```python
from build123d import *

# Parameters (mm, degrees)
F0_W     = 151.8794447184
F0_H     = 152.5772064924
F1_DEPTH = 4.318
F2_W     = 130.1674246788
F2_H     = 5.3557232022
F2_H_2   = 7.4514448643
F3_DEPTH = 5.588
F4_W     = 51.2286853045
F4_H     = 29.5729218051
F5_DEPTH = 23.876


with BuildPart() as f1:
    # F0 (on Top) → F1 (new body)
    with BuildSketch(Plane.XY):
        with Locations((0.1162961125, 0)):
            Rectangle(F0_W, F0_H)
    extrude(amount=F1_DEPTH)

    # F2 (on face) → F3 (join)
    with BuildSketch(Plane.XY.offset(4.318)):
        Polygon((-65.2001425624, 63.5701417923), (-65.2001425624, 68.9258649945), (-71.2544471025, 68.9258649945), (-71.2544471025, -70.7887262106), (-65.2001425624, -70.7887262106), (-65.2001425624, -70.5558732152), (-65.2001425624, -63.1044283509), align=None)
        with Locations((-0.116430223, 66.2480033934)):
            Rectangle(F2_W, F2_H)
        Polygon((73.8158747554, 68.9258649945), (64.9672821164, 68.9258649945), (64.9672821164, 63.5701417923), (64.9672821164, -63.1044283509), (64.9672821164, -70.5558732152), (73.8158747554, -70.5558732152), align=None)
        with Locations((-0.116430223, -66.8301507831)):
            Rectangle(F2_W, F2_H_2)
    extrude(amount=F3_DEPTH)

    # F4 (on face) → F5 (join)
    with BuildSketch(Plane.XY.offset(4.318)):
        with Locations((2.0957188681, 10.8278808184)):
            Rectangle(F4_W, F4_H)
    extrude(amount=F5_DEPTH)


solid = f1.part
```
Input: part model. Units: mm. Frame: model coordinates. A direction names the side the tool comes from. Coordinates: 2 decimals unless noted, no trailing zeros. Write each loop counter-clockwise with the first axis right and the second up, starting at its lowest first coordinate (ties: lowest second). Pieces come first, ordered by that corner, then holes.
1) Section B-B on x = 13. Output: boundary loops of the cut face in (y, z).
2) Section A-A on y = 0. Output: boundary loops of the cut face in (x, z).
3) Pin query (flat end, axial travel): pin 1 Ø5 at (x, y) = (-36.5, 31.5) entering from +Z; pin 2 Ø10 at (x, z) = (52.5, 12.5) entering from +Y; pin 3 Ø1.7 at (x, z) = (-68, 8.5) entering from -Y; pin 4 Ø1.5 at (x, y) = (-60.5, -1.5) entering from -Z. Return the tip coordinate at first contact, or that it passes through.
4) Section C-C on z = 19.25. Output: boundary loops of the cut face in (x, y), and give its area (3 significant figures).
5) Set-up query: faces 5 (the flat face through (73.816, -2, 7)), 6 (the flat face through (2, 68.926, 7)), 7 (the flat face through (-71.254, 0, 7)), 8 (the flat face through (64.967, 1, 7)). Return all of +Z, -Z, +X, -X, +Y, -Y with unobstructed straight access to the full face (end or side cutting, diameter ignored); none if empty.
6) Section D-D on y = 36. Output: boundary loops of the cut face in (x, z).
7) Mould query, pull axis X, two halves, no side actions, for faces 1 (the flat face through (-1, 63.57, 7)), 2 (the flat face through (-75.823, -1, 2)), 3 (the flat face through (-1, 1, 0)), 4 (the flat face through (-23.519, 11, 16)). Classes: pulls with the +X half, pulls with the -X half, needs draft (parallel to the pull), parting line crosses it, or undercut.
8) Material intervals for line 1 along X through (y, z) = (24, 9); line 2 along Y through (x, z) = (-7, 4.5); line 3 along X through (y, z) = (30, 6), sorted ascending.
Check result:
1. outline: (-76.29, 0) - (76.29, 0) - (76.29, 4.32) - (68.93, 4.32) - (68.93, 9.91) - (63.57, 9.91) - (63.57, 4.32) - (25.61, 4.32) - (25.61, 28.19) - (-3.96, 28.19) - (-3.96, 4.32) - (-63.1, 4.32) - (-63.1, 9.91) - (-70.56, 9.91) - (-70.56, 4.32) - (-76.29, 4.32) - close
2. outline: (-75.82, 0) - (76.06, 0) - (76.06, 4.32) - (73.82, 4.32) - (73.82, 9.91) - (64.97, 9.91) - (64.97, 4.32) - (27.71, 4.32) - (27.71, 28.19) - (-23.52, 28.19) - (-23.52, 4.32) - (-65.2, 4.32) - (-65.2, 9.91) - (-71.25, 9.91) - (-71.25, 4.32) - (-75.82, 4.32) - close
3. pin 1: stops at z = 4.32
3. pin 2: stops at y = 68.93
3. pin 3: stops at y = -70.79
3. pin 4: stops at z = 0
4. outline: (-23.52, -3.96) - (27.71, -3.96) - (27.71, 25.61) - (-23.52, 25.61) - close
4. area: 1,510 mm2
5. face 5: +Z, +X, +Y, -Y
5. face 6: +Z, +X, -X, +Y
5. face 7: +Z, -X, +Y, -Y
5. face 8: +Z
6. outline: (-75.82, 0) - (76.06, 0) - (76.06, 4.32) - (73.82, 4.32) - (73.82, 9.91) - (64.97, 9.91) - (64.97, 4.32) - (-65.2, 4.32) - (-65.2, 9.91) - (-71.25, 9.91) - (-71.25, 4.32) - (-75.82, 4.32) - close
7. face 1: undercut
7. face 2: pulls with the -X half
7. face 3: needs draft
7. face 4: undercut
8. line 1: x = -71.25 to -65.2, -23.52 to 27.71, 64.97 to 73.82
8. line 2: y = -70.56 to -63.1, -3.96 to 25.61, 63.57 to 68.93
8. line 3: x = -71.25 to -65.2, 64.97 to 73.82
